For this review, take the finished solid that the model builds, in its own axes (mm). A direction names the side the tool comes from. Round coordinates to 2 decimals unless told otherwise and drop trailing zeros. Loops run counter-clockwise (first coordinate to the right, second up) from the corner with the lowest first, then second, coordinate; pieces in that order, holes last. Notation, with made-up numbers: (12, 14.25) -> (64, 14.25) arc R36 cw to (64, 49.25) -> close; hole circle Ø2 at (64.5, 45.25). An arc over 180 degrees is marked (long way). Write each question's results on one line, items separated by ' | '.
```python
from build123d import *

# Parameters (mm, degrees)
SKETCH1_R               = 2.25
BOSS_EXTRUDE1_DEPTH     = 6.5
CUT_EXTRUDE1_DEPTH      = 5
CUT_EXTRUDE1_DEPTH_BACK = 5
SKETCH2_W               = 33
SKETCH2_H               = 3.25
SKETCH2_W_2             = 54
FILLET1_R               = 5


with BuildPart() as part:
    # Sketch1 → Boss-Extrude1 (new body)
    with BuildSketch(Plane(origin=(0, 0, 0), x_dir=(1, 0, 0), z_dir=(0, 1, 0))):
        Polygon((0, 0), (-5, 0), (-5, 90), (5, 90), (5, 0), align=None)
        with Locations(Location((0, 20, 0), (0, 0, 90))):
            Circle(SKETCH1_R, mode=Mode.SUBTRACT)
        with Locations(Location((0, 5, 0), (0, 0, 90))):
            Circle(SKETCH1_R, mode=Mode.SUBTRACT)
        with Locations(Location((0, 80, 0), (0, 0, 90))):
            Circle(SKETCH1_R, mode=Mode.SUBTRACT)
    extrude(amount=BOSS_EXTRUDE1_DEPTH)

    # Sketch2 → Cut-Extrude1 (cut, two sides: drawn at the far end of the back side and taken through both)
    with BuildSketch(Plane(origin=(0, 0, 0), x_dir=(0, 0, -1), z_dir=(1, 0, 0)).offset(-CUT_EXTRUDE1_DEPTH_BACK)):
        with Locations((16.5, 1.625)):
            Rectangle(SKETCH2_W, SKETCH2_H)
        with Locations((63, 4.875)):
            Rectangle(SKETCH2_W_2, SKETCH2_H)
    extrude(amount=CUT_EXTRUDE1_DEPTH + CUT_EXTRUDE1_DEPTH_BACK, mode=Mode.SUBTRACT)

    # Fillet1
    # the kernel refuses this fillet: 5 mm, written as the material it adds along each edge
    with BuildSketch(Plane(origin=(5, 3.25, -33), x_dir=(0, 0, 1), z_dir=(-1, 0, 0))) as fillet1_piece_1:
        with BuildLine():
            CenterArc((4.683748499, -5), FILLET1_R, 90, 69.512684885)
            Line((0, -3.25), (-0.09367497, -3.215))
            ThreePointArc((-0.09367497, -3.215), (-0.1, -1.625), (-0.1, 0))
            Line((-0.1, 0), (0, 0.1))
            Line((0, 0.1), (4.683748499, 0.1))
            Line((4.683748499, 0.1), (4.683748499, 0))
        make_face()
    extrude(amount=10)
    with BuildSketch(Plane(origin=(-5, 3.25, -36), x_dir=(0, 0, -1), z_dir=(1, 0, 0))) as fillet1_piece_2:
        with BuildLine():
            CenterArc((4.683748499, 5), FILLET1_R, 200.487315115, 69.512684885)
            Line((0, 3.25), (-0.09367497, 3.215))
            ThreePointArc((-0.09367497, 3.215), (-0.1, 1.625), (-0.1, 0))
            Line((-0.1, 0), (0, -0.1))
            Line((0, -0.1), (4.683748499, -0.1))
            Line((4.683748499, -0.1), (4.683748499, 0))
        make_face()
    extrude(amount=10)


solid = part.part
```
1. Draft analysis for pull direction Z (two halves, no side actions). For faces 1 (the face through (0, 5, 0)), 2 (the face through (-0.676, 4.852, -7.146)), 3 (the face through (0, 3.25, -65)), state which applies: released by +Z, released by -Z, zero draft, split by the parting line, or undercut.
Values found:
face 1: released by +Z | face 2: undercut | face 3: zero draft
2. To check wall thickness, follow probe 1 along X at (y, z) = (4.9, -20); probe 2 along Z at (x, y) = (-1.25, 5.5); probe 3 along Z at (x, y) = (-0.75, 6). State the ranges of each line that lie inside material, in increasing order.
Values found:
probe 1: x = -5 to -2.25, 2.25 to 5 | probe 2: z = -36.51 to -21.87, -18.13 to -6.87, -3.13 to 0 | probe 3: z = -36.22 to -22.12, -17.88 to -7.12, -2.88 to 0
3. Consider section A-A (z = -20). State the section outline as (x, y) points.
Values found:
outline: (-5, 3.25) -> (-2.25, 3.25) -> (-2.25, 6.5) -> (-5, 6.5) -> close; (2.25, 3.25) -> (5, 3.25) -> (5, 6.5) -> (2.25, 6.5) -> close
4. Tool access review of faces 4 (the face through (0, 3.25, -14)), 5 (the face through (0, 2, -90)): name each direction out of +Z, -Z, +X, -X, +Y, -Y from which nothing blocks a thin tool from reaching the whole face with its end or side.
Values found:
face 4: +Z, +X, -X, -Y | face 5: -Z, +X, -X, +Y, -Y
5. For pin 1 (2 mm diameter, centred on x = -1, z = -48.5, fed in from +Y); pin 2 (5 mm diameter, centred on x = 0, z = -5, fed in from -Y); pin 3 (1 mm diameter, centred on x = -1.5, y = 1, fed in from +Z); pin 4 (3.5 mm diameter, centred on x = 0, z = -80, fed in from -Y), all flat-tipped, find the tip position at first contact; note any pin that passes through.
Values found:
pin 1: stops at y = 3.25 | pin 2: stops at y = 3.25 | pin 3: stops at z = -32.12 | pin 4: passes through
6. Consider section D-D (y = 5.5). State the section outline as (x, z) points.
Values found:
outline: (-5, -36.51) -> (5, -36.51) -> (5, 0) -> (-5, 0) -> close; hole circle Ø4.5 at (0, -20); hole circle Ø4.5 at (0, -5)
7. Consider section B-B (x = 1.25). State the section outline as (y, z) points, plus the area to 3 significant figures.
Values found:
outline: (0, -90) -> (3.25, -90) -> (3.25, -81.87) -> (0, -81.87) -> close; (0, -78.13) -> (3.25, -78.13) -> (3.25, -40.68) arc R5 cw to (6.5, -36) -> (6.5, -21.87) -> (3.25, -21.87) -> (3.25, -28.32) arc R5 cw to (0, -33) -> close; (3.25, -18.13) -> (6.5, -18.13) -> (6.5, -6.87) -> (3.25, -6.87) -> close; (3.25, -3.13) -> (6.5, -3.13) -> (6.5, 0) -> (3.25, 0) -> close | area: 274 mm2
8. Consider section C-C (y = 1.75). State the section outline as (x, z) points, plus the area to 3 significant figures.
Values found:
outline: (-5, -90) -> (5, -90) -> (5, -31.89) -> (-5, -31.89) -> close; hole circle Ø4.5 at (0, -80) | area: 565 mm2
